Can you work these out from the model? Positions are in its coordinate system, mm. A direction names the side the tool comes from. Coordinates: 2 decimals unless noted, no trailing zeros. Order: outer loops, then holes, each group sorted by start corner. A loop starts at its lowest first (then second) coordinate and runs counter-clockwise, first axis right, second up. Notation, with made-up numbers: (14, -37.5) -> (37, -37.5) arc R29 ccw to (37, 0.5) -> close; hole circle Ø4 at (66, 43.25). An arc over 180 degrees is marked (long way). Answer in a Markdown table with one row per item. Add a question column.
1. On a 3-axis mill with a long thin cutter (end or side, diameter ignored), from which of +Z, -Z, +X, -X, +Y, -Y can I reach the whole of each face in a straight line? I mean faces 1 (the face through (-3.896, 0.171, 5.253)), 2 (the face through (-0.1, 0, 8)), 3 (the face through (-1, 0, 9.9)). Say none if no direction works.
2. Will these pins go through, and if not, where does the flat tip stop? pin 1 (6 mm diameter, centred on x = -7.5, y = -7.5, fed in from +Z); pin 2 (1 mm diameter, centred on x = 1.5, y = 0, fed in from +Z).
3. Imagine slicing it at A-A on z = 4.75. Write out the boundary of the cut face in (x, y), plus the area to 3 significant figures.
4. Imagine slicing it at B-B on z = 8.5. Write out the boundary of the cut face in (x, y).
5. If I drill on line 1 along Z through (x, y) = (6.5, 3.25); line 2 along X through (y, z) = (-0.25, 6.5); line 3 along Y through (x, z) = (8.25, 0.5), over which ranges is the centre line in solid material (lowest first)? Write a range as [from, to].
from build123d import *

# Parameters (mm, degrees)
F0_R        = 10
F1_DEPTH    = 2
F2_R        = 4.5
F3_DEPTH    = 1
F4_R        = 3.9
F5_DEPTH    = 6.9
F8_DEPTH    = 5.5
F9_T8_ANGLE = 250.6318620022
F10_R       = 0.4


# Not quite as in the source:
# - a fillet or chamfer that OpenCascade refuses, or shapes differently, is made with other operations: its cross-section is extruded or revolved along the edge and cut away or added


with BuildPart() as f1:
    # F0 (on Top) → F1 (new body)
    with BuildSketch(Plane.XY):
        Circle(F0_R)
    extrude(amount=F1_DEPTH)

    # F2 (on face) → F3 (join)
    with BuildSketch(Plane.XY.offset(2)):
        Circle(F2_R)
    extrude(amount=F3_DEPTH)

    # F4 (on face) → F5 (join)
    with BuildSketch(Plane.XY.offset(3)):
        Circle(F4_R)
    extrude(amount=F5_DEPTH)

    # F7 (on offset) → F8 (cut, symmetric)
    with BuildSketch(Plane.XY.offset(10.9)):
        Polygon((5.1383636892, 5.7038869709), (-0.1, 5.7038869709), (-0.1, -5.6052659638), (5.1383636892, -5.3080837242), align=None)
    extrude(amount=F8_DEPTH, both=True, mode=Mode.SUBTRACT)

    # F9: fillet of radius 1 on 4 edges, made by hand

    # F9_s1 → F9_t2 (revolve, cut)
    with BuildSketch(Plane.XZ):
        with BuildLine():
            ThreePointArc((10, 1), (9.7071067812, 0.2928932188), (9, 0))
            Line((9, 0), (10, 0))
            Line((10, 0), (10, 1))
        make_face()
    revolve(axis=Axis((0, 0, 0), (0, 0, 1)), mode=Mode.SUBTRACT)

    # F9_s3 → F9_t4 (revolve, cut)
    with BuildSketch(Plane.XZ):
        with BuildLine():
            ThreePointArc((10, 1), (9.7071067812, 1.7071067812), (9, 2))
            Line((9, 2), (10, 2))
            Line((10, 2), (10, 1))
        make_face()
    revolve(axis=Axis((0, 0, 2), (0, 0, 1)), mode=Mode.SUBTRACT)

    # F9_s5 → F9_t6 (revolve, cut)
    with BuildSketch(Plane.XZ):
        with BuildLine():
            ThreePointArc((4.5, 2.083484861), (4.3366600265, 2.6312074185), (3.9, 3))
            Line((3.9, 3), (4.5, 3))
            Line((4.5, 3), (4.5, 2.083484861))
        make_face()
    revolve(axis=Axis((0, 0, 3), (0, 0, 1)), mode=Mode.SUBTRACT)

    # F9_s7 → F9_t8 (revolve, cut)
    with BuildSketch(Plane(origin=(0, 0, 0), x_dir=(0, 0, 1), z_dir=(0.8159768861, -0.5780845278, 0))):
        with BuildLine():
            ThreePointArc((8.9, -3.9), (9.6071067812, -3.6071067812), (9.9, -2.9))
            Line((9.9, -2.9), (9.9, -3.9))
            Line((9.9, -3.9), (8.9, -3.9))
        make_face()
    revolve(axis=Axis((0, 0, 9.9), (0, 0, 1)), revolution_arc=F9_T8_ANGLE, mode=Mode.SUBTRACT)

    # F10
    f10_edges = [f1.edges().sort_by_distance(p)[0] for p in [
        (-0.1, -3.898718, 7.15),
        (-0.1, 3.898718, 7.15),
        (-0.1, 3.605629, 9.607198),
        (-0.1, -3.605629, 9.607198),
        (-0.1, 0, 9.9),
        (2.722132, -2.792848, 5.4),
        (2.722132, 2.792848, 5.4),
        (-0.1, 0, 5.4),
    ]]
    fillet(f10_edges, radius=F10_R)


solid = f1.part
Answers follow:
| question | item | result |
|---|---|---|
| 1 | face 1 | +Z |
| 1 | face 2 | +Z, +X, +Y, -Y |
| 1 | face 3 | +Z, +X, -X, +Y, -Y |
| 2 | pin 1 | stops at z = 2 |
| 2 | pin 2 | stops at z = 5.4 |
| 3 | outline | circle Ø7.8 at (0, 0) |
| 3 | area | 47.8 mm² |
| 4 | outline | (-0.56, -3.86) arc R0.4 ccw to (-0.1, -3.46) -> (-0.1, 3.46) arc R0.4 ccw to (-0.56, 3.86) arc R3.9 ccw to start |
| 5 | line 1 | z = [0, 2] |
| 5 | line 2 | x = [-3.89, -0.1] |
| 5 | line 3 | y = [-5.41, 5.41] |
